Read the model definition and answer for the solid it produces. Units are mm, in the model's axes. Coordinates: 2 decimals unless noted, no trailing zeros. Write each loop counter-clockwise with the first axis right and the second up, starting at its lowest first coordinate (ties: lowest second). Pieces come first, ordered by that corner, then holes.
1) The part is cut by section A-A (y = 15). Determine the outline of the cut face in (x, z).
2) Find the intervals of material crossed by line 1 (X direction, y = 42, z = 0.05); line 2 (Z direction, x = 0.15, y = 19); line 3 (Z direction, x = -0.8, y = 10.5), in increasing order.
3) The part is cut by section B-B (x = -0.45). Determine the outline of the cut face in (y, z).
4) The part is cut by section C-C (z = -0.4). Determine the outline of the cut face in (x, y), then the cut area to 3 significant figures.
Autodesk Inventor part; units mm, degrees
ref_plane "YZ Plane" through (0, 0, 0) normal (1, 0, 0) x (0, 1, 0)
ref_plane "XZ Plane" through (0, 0, 0) normal (0, 1, 0) x (-1, 0, 0)
ref_plane "XY Plane" through (0, 0, 0) normal (0, 0, 1) x (1, 0, 0)
sketch "Sketch1" plane through (0, 0, 0) normal (0, 1, 0) x (-1, 0, 0)
  circle A0 centre (0, 0) radius 1
  dimension "d0" = 2
extrude "Extrusion1" add sketch "Sketch1" along normal blind 55
move faces "Move1" translate (0, -2.5, 0) faces at (-0.5848, 55, -0.397)
move faces "Move2" translate (0, -0.002, 0) faces at (-0.2495, 52.5, 0.221)
properties part number "LOOP1_COLL_L"
Reported:
1. outline: circle Ø2 at (0, 0)
2. line 1: x = -1 to 1
2. line 2: z = -0.99 to 0.99
2. line 3: z = -0.6 to 0.6
3. outline: (0, -0.89) - (52.5, -0.89) - (52.5, 0.89) - (0, 0.89) - close
4. outline: (-0.92, 0) - (0.92, 0) - (0.92, 52.5) - (-0.92, 52.5) - close
4. area: 96.2 mm2
